from build123d import *

# Parameters (mm, degrees)
SKETCH1_R           = 10
BOSS_EXTRUDE1_DEPTH = 2
SKETCH2_R           = 7.5
BOSS_EXTRUDE2_DEPTH = 8
CUT_EXTRUDE2_REACH  = 19.321


with BuildPart() as part:
    # Sketch1 → Boss-Extrude1 (new body)
    with BuildSketch(Plane(origin=(0, 0, 0), x_dir=(1, 0, 0), z_dir=(0, 1, 0))):
        with Locations(Location((0, 0, 0), (0, 0, 270))):
            Circle(SKETCH1_R)
    extrude(amount=BOSS_EXTRUDE1_DEPTH)

    # Sketch2 → Boss-Extrude2 (add)
    with BuildSketch(Plane(origin=(0, 2, 0), x_dir=(1, 0, 0), z_dir=(0, 1, 0))):
        with Locations(Location((0, 0, 0), (0, 0, 270))):
            Circle(SKETCH2_R)
    extrude(amount=BOSS_EXTRUDE2_DEPTH)

    # Sketch4 → Cut-Extrude2 (cut, up to next)
    with BuildSketch(Plane(origin=(0, 10, 0), x_dir=(1, 0, 0), z_dir=(0, 1, 0)), mode=Mode.PRIVATE) as cut_extrude2_sk1:
        Polygon((2.5, 1.443375673), (0, 2.886751346), (-2.5, 1.443375673), (-2.5, -1.443375673), (0, -2.886751346), (2.5, -1.443375673), align=None)
    cut_extrude2_tool1 = extrude(cut_extrude2_sk1.sketch, amount=-CUT_EXTRUDE2_REACH, mode=Mode.PRIVATE) & part.part
    add(cut_extrude2_tool1.solids().sort_by_distance((0, 10, 0))[0], mode=Mode.SUBTRACT)


solid = part.part
Design review of the part built by this model. Coordinates are the model's own, in mm. A direction names the side the tool comes from. Coordinates: 2 decimals unless noted, no trailing zeros. Loops run counter-clockwise (first coordinate to the right, second up) from the corner with the lowest first, then second, coordinate; pieces in that order, holes last. Notation, with made-up numbers: (18, 13) -> (30, 13) arc R14 cw to (30, 30) -> close; hole circle Ø3 at (42, 42.25). An arc over 180 degrees is marked (long way). Use a Markdown table: item, result. Add a question column.
Item 1: We need section B-B, the plane y = 3.25. Write out the cut boundary in (x, z).
Item 2: We need section D-D, the plane x = 6.75. Write out the cut boundary in (y, z), and give its area (3 significant figures).
Item 3: We need section A-A, the plane z = 0. Write out the cut boundary in (x, y), and give its area (3 significant figures).
Item 4: Machinability: for faces 5 (the flat face through (-1.233, 5.07, -2.175)), 6 (the flat face through (-2, 0, 2)), 7 (the cylindrical face through (0.33, 5.944, -7.493)), which of the approach directions +Z, -Z, +X, -X, +Y, -Y give a long, thin tool a straight path to every point of the face, cutting with its end or side? Answer none if there is none.
Item 5: We need section C-C, the plane x = 0.5. Write out the cut boundary in (y, z).
Item 6: Clearance check with flat-ended pins moving along their axes: P1, Ø1.5, axis at x = -7.5, y = 8, coming from the +Z side; P2, Ø4, axis at x = 3.5, y = 6, coming from the +Z side; P3, Ø0.9, axis at y = 4, z = 0, coming from the +X side; P4, Ø2, axis at x = -1, z = -1, coming from the -Y side. State where each tip first meets the part, or that it passes through.
Item 7: The part is to be moulded in two halves that separate along Z. For faces 1 (the cylindrical face through (-9.76, 0.99, -2.17)), 2 (the flat face through (1.233, 5.07, 2.175)), 3 (the flat face through (-1.267, 5.07, 2.155)), 4 (the flat face through (0.1, 10, 3.2)), say which applies: +Z half, -Z half, draft (parallel to the pull), parting line (faces both ways), or undercut.
Item 8: Wall thickness on L1, parallel to Y at x = -8, z = 1.75; L2, parallel to X at y = 4.5, z = 2.5; L3, parallel to Z at x = -2, y = 4.75: over which ranges is each line inside the solid? List them lowest first. Write a range as from..to.
Numbers:
| question | item | result |
|---|---|---|
| 1 | outline | circle Ø15 at (0, 0); hole (-2.5, -1.44) -> (0, -2.89) -> (2.5, -1.44) -> (2.5, 1.44) -> (0, 2.89) -> (-2.5, 1.44) -> close |
| 2 | outline | (0, -7.38) -> (2, -7.38) -> (2, -3.27) -> (10, -3.27) -> (10, 3.27) -> (2, 3.27) -> (2, 7.38) -> (0, 7.38) -> close |
| 2 | area | 81.8 mm^2 |
| 3 | outline | (-10, 0) -> (-2.5, 0) -> (-2.5, 10) -> (-7.5, 10) -> (-7.5, 2) -> (-10, 2) -> close; (2.5, 0) -> (10, 0) -> (10, 2) -> (7.5, 2) -> (7.5, 10) -> (2.5, 10) -> close |
| 3 | area | 110 mm^2 |
| 4 | face 5 | +Y, -Y |
| 4 | face 6 | +Z, -Z, +X, -X, -Y |
| 4 | face 7 | +Y |
| 5 | outline | (0, -9.99) -> (2, -9.99) -> (2, -7.48) -> (10, -7.48) -> (10, -2.6) -> (0, -2.6) -> close; (0, 2.6) -> (10, 2.6) -> (10, 7.48) -> (2, 7.48) -> (2, 9.99) -> (0, 9.99) -> close |
| 6 | P1 | stops at z = 3.27 |
| 6 | P2 | stops at z = 7.35 |
| 6 | P3 | stops at x = 7.5 |
| 6 | P4 | passes through |
| 7 | face 1 | parting line |
| 7 | face 2 | undercut |
| 7 | face 3 | undercut |
| 7 | face 4 | draft |
| 8 | L1 | y = 0..2 |
| 8 | L2 | x = -7.07..-0.67, 0.67..7.07 |
| 8 | L3 | z = -7.23..-1.73, 1.73..7.23 |
